Input: part model. Units: mm. Frame: model coordinates. A direction names the side the tool comes from. Coordinates: 2 decimals unless noted, no trailing zeros. Order: outer loops, then holes, each group sorted by start corner. A loop starts at its lowest first (then second) coordinate and runs counter-clockwise, first axis right, second up. Notation, with made-up numbers: (-8, -24.5) -> (22, -24.5) arc R28 cw to (22, 11.5) -> close; hole circle Ø3 at (17, 80). An arc over 180 degrees is marked (long way). One line per question, with ' | ' between items.
```python
from build123d import *

# Parameters (mm, degrees)
F2_DEPTH = 2
F0_R     = 2.5
F3_DEPTH = 3
F4_COUNT = 6
F5_DEPTH = 3


with BuildPart() as f2:
    # F0 (on Top) → F2 (new body)
    with BuildSketch(Plane.XY):
        with BuildLine():
            Line((-16.25, 1), (-17.4714052097, 1))
            ThreePointArc((-17.4714052097, 1), (-17.4769180723, 0.8985180536), (-17.4818414863, 0.7970058027))
            ThreePointArc((-17.4818414863, 0.7970058027), (-17.4954597826, 0.3986063162), (-17.5, 0))
            ThreePointArc((-17.5, 0), (-17.4928498417, -0.5002043737), (-17.4714052097, -1))
            Line((-17.4714052097, -1), (-16.25, -1))
            Line((-16.25, -1), (-16.25, 1))
        make_face()
    extrude(amount=F2_DEPTH)

    # F0 (on Top) → F3 (join)
    with BuildSketch(Plane.XY):
        with BuildLine():
            ThreePointArc((-17.4714052097, -1), (0.5002043737, -17.4928498417), (17.5, 0))
            ThreePointArc((17.5, 0), (0.5002043737, 17.4928498417), (-17.4714052097, 1))
            Line((-17.4714052097, 1), (-16.25, 1))
            Line((-16.25, 1), (-16.25, -1))
            Line((-16.25, -1), (-17.4714052097, -1))
        make_face()
        with Locations((0, -12.5)):
            Circle(F0_R, mode=Mode.SUBTRACT)
        with Locations((0, 12.5)):
            Circle(F0_R, mode=Mode.SUBTRACT)
        with BuildLine():
            Line((-16.25, 1), (-17.4714052097, 1))
            ThreePointArc((-17.4714052097, 1), (-17.4769180723, 0.8985180536), (-17.4818414863, 0.7970058027))
            ThreePointArc((-17.4818414863, 0.7970058027), (-17.4954597826, 0.3986063162), (-17.5, 0))
            ThreePointArc((-17.5, 0), (-17.4928498417, -0.5002043737), (-17.4714052097, -1))
            Line((-17.4714052097, -1), (-16.25, -1))
            Line((-16.25, -1), (-16.25, 1))
        make_face()
    extrude(amount=-F3_DEPTH)

    # F4: F2 ×6 about axis
    f4_axis = Axis((0, 0, 0), (0, 0, 1))


with BuildPart() as f2_1:
    add(f2.part)
    for i in range(1, F4_COUNT):
        add(f2.part.rotate(f4_axis, i * 360 / F4_COUNT))

    # F0 (on Top) → F5 (cut, through all)
    with BuildSketch(Plane.XY):
        with Locations((0, -12.5)):
            Circle(F0_R)
        with Locations((0, 12.5)):
            Circle(F0_R)
    extrude(amount=-F5_DEPTH, mode=Mode.SUBTRACT)


solid = f2_1.part
```
1. Cut plane A-A, the plane x = 0. Return loops of the section in (y, z).
Recorded:
outline: (-17.5, -3) -> (-15, -3) -> (-15, 0) -> (-17.5, 0) -> close; (-10, -3) -> (10, -3) -> (10, 0) -> (-10, 0) -> close; (15, -3) -> (17.5, -3) -> (17.5, 0) -> (15, 0) -> close
2. Pin query (flat end, axial travel): pin 1 Ø0.6 at (x, z) = (-17, 1) entering from -Y; pin 2 Ø2 at (x, y) = (-7.5, 13) entering from +Z; pin 3 Ø1.3 at (x, z) = (17, 1) entering from +Y. Return the tip coordinate at first contact, or that it passes through.
Recorded:
pin 1: stops at y = -1 | pin 2: stops at z = 0 | pin 3: stops at y = 1
3. Cut plane D-D, the plane y = -2. Return loops of the section in (x, z), and give its area (3 significant figures).
Recorded:
outline: (-17.39, -3) -> (17.39, -3) -> (17.39, 0) -> (-17.39, 0) -> close | area: 104 mm^2
4. Cut plane C-C, the plane y = -12.5. Return loops of the section in (x, z).
Recorded:
outline: (-12.25, -3) -> (-2.5, -3) -> (-2.5, 0) -> (-12.25, 0) -> close; (2.5, -3) -> (12.25, -3) -> (12.25, 0) -> (2.5, 0) -> close
5. Access query for faces 4 (the face through (7.56, -15.094, 0.986)), 5 (the face through (-8.11, -14.08, 0.99)), 6 (the face through (-7.56, 15.094, 0.986)), 7 (the face through (17, -1, 1)). Directions: +Z, -Z, +X, -X, +Y, -Y. A direction counts if a zero-diameter tool reaches every point of the face in a straight line with its end or side. Return the directions, or none.
Recorded:
face 4: +Z, -Y | face 5: +Z | face 6: +Z, +Y | face 7: +Z, +X, -X, -Y
6. Mould query, pull axis X, two halves, no side actions, for faces 1 (the face through (-8, -15, 2)), 2 (the face through (9.3, -14.11, 0.99)), 3 (the face through (-8.137, 14.066, 0.986)). Classes: released by +X, released by -X, zero draft, split by the parting line, or undercut.
Recorded:
face 1: zero draft | face 2: released by +X | face 3: undercut
7. Ray query, line 1 (Y direction, x = 0, z = -2.2); line 2 (Y direction, x = 2, z = -0.3); line 3 (Z direction, x = 13, y = -2). Return the intervals inside material, ascending. Write a range as [from, to].
Recorded:
line 1: y = [-17.5, -15], [-10, 10], [15, 17.5] | line 2: y = [-17.39, -14], [-11, 11], [14, 17.39] | line 3: z = [-3, 0]
8. Cut plane B-B, the plane z = -1.15. Return loops of the section in (x, y).
Recorded:
outline: (-17.48, 0.8) arc R17.5 ccw to (-9.6, -14.63) arc R17.5 ccw to (-9.43, -14.74) arc R17.5 ccw to (7.87, -15.63) arc R17.5 ccw to (8.05, -15.54) arc R17.5 ccw to (17.47, -1) arc R17.5 ccw to (17.48, -0.8) arc R17.5 ccw to (9.6, 14.63) arc R17.5 ccw to (9.43, 14.74) arc R17.5 ccw to (-7.87, 15.63) arc R17.5 ccw to (-8.05, 15.54) arc R17.5 ccw to (-17.47, 1) arc R17.5 ccw to start; hole circle Ø5 at (0, -12.5); hole circle Ø5 at (0, 12.5)
